The listing builds one solid part. Answer for the finished solid, in the listing's coordinates (mm). Give positions to 0.01 mm unless a question says otherwise; leave off trailing zeros. Loops run counter-clockwise (first coordinate to the right, second up) from the corner with the lowest first, then second, coordinate; pieces in that order, holes last. Notation, with made-up numbers: (42, 10) - (46, 10) arc R25 ccw to (46, 25) - close; hole circle Ø7 at (-34.75, -22). An arc over 180 degrees is marked (long way). Write each question's results on one line, items separated by ' | '.
from build123d import *
from build123d.topology import SkipClean

# Parameters (mm, degrees)
SKETCH1_R           = 2.98
BOSS_EXTRUDE1_DEPTH = 5.55
SKETCH2_R           = 2.5
CUT_EXTRUDE1_DEPTH  = 4.9
SKETCH3_R           = 1.44
CUT_EXTRUDE2_DEPTH  = 7.968737332
CHAMFER1_SIZE       = 0.25
THREAD1_PITCH       = 0.8


with BuildPart() as part:
    # Sketch1 → Boss-Extrude1 (new body)
    with BuildSketch(Plane(origin=(0, 0, 0), x_dir=(1, 0, 0), z_dir=(0, 1, 0))):
        with Locations(Location((0, 0, 0), (0, 0, 270))):
            Circle(SKETCH1_R)
    extrude(amount=BOSS_EXTRUDE1_DEPTH)

    # Sketch2 → Cut-Extrude1 (cut)
    with BuildSketch(Plane.XZ):
        with Locations(Location((0, 0, 0), (0, 0, 270))):
            Circle(SKETCH2_R)
    extrude(amount=-CUT_EXTRUDE1_DEPTH, mode=Mode.SUBTRACT)

    # Sketch3 → Cut-Extrude2 (cut, through all)
    with BuildSketch(Plane(origin=(0, 5.55, 0), x_dir=(1, 0, 0), z_dir=(0, 1, 0))):
        with Locations(Location((0, 0, 0), (0, 0, 270))):
            Circle(SKETCH3_R)
    extrude(amount=-CUT_EXTRUDE2_DEPTH, mode=Mode.SUBTRACT)

    # Chamfer1
    chamfer1_edges = [part.edges().sort_by_distance(p)[0] for p in [
        (0, 5.55, -2.98),
    ]]
    chamfer(chamfer1_edges, length=CHAMFER1_SIZE)

    # Thread1: the profile of Thread Profile1 profile screwed along a right-hand helix of 2.5 turns, 8 arcs to a turn; built about Z, then put on its axis
    with SkipClean():  # the faces are left unmerged after this step: merging them gives an invalid solid
        thread1_z = Axis((0, 0, 0), (0, 0, 1))
        thread1_corners = [(2.4997, 0, -0.000173205), (2.9330127, 0, 0.249999999), (2.9330127, 0, 0.349999999), (2.4997, 0, 0.600173203)]
        with BuildLine(mode=Mode.PRIVATE) as thread1_profile:
            Line(thread1_corners[0], thread1_corners[1])
            Line(thread1_corners[1], thread1_corners[2])
            Line(thread1_corners[2], thread1_corners[3])
            Line(thread1_corners[3], thread1_corners[0])
        thread1_cap = Face(thread1_profile.wire())
        thread1_turn_angles = [0, 22.5, 45, 67.5, 90, 112.5, 135, 157.5, 180, 202.5, 225, 247.5, 270, 292.5, 315, 337.5, 360]
        thread1_turn_weights = [1, 0.9238795325112867, 1, 0.9238795325112867, 1, 0.9238795325112867, 1, 0.9238795325112867, 1, 0.9238795325112867, 1, 0.9238795325112867, 1, 0.9238795325112867, 1, 0.9238795325112867, 1]
        thread1_turn_rails = [Edge.make_bspline([Vector(p[0], p[1], 0).rotate(thread1_z, thread1_turn_angles[k]) / thread1_turn_weights[k] + Vector(0, 0, p[2] + THREAD1_PITCH * thread1_turn_angles[k] / 360) for k in range(17)], [0, 0, 0, 1, 1, 2, 2, 3, 3, 4, 4, 5, 5, 6, 6, 7, 7, 8, 8, 8], 2, thread1_turn_weights) for p in thread1_corners]
        thread1_turn_sides = [Face.make_surface_from_curves(thread1_turn_rails[p[0]], thread1_turn_rails[p[1]]) for p in [(0, 1), (1, 2), (2, 3), (3, 0)]]
        thread1_last_angles = [720, 742.5, 765, 787.5, 810, 832.5, 855, 877.5, 900]
        thread1_last_weights = [1, 0.9238795325112867, 1, 0.9238795325112867, 1, 0.9238795325112867, 1, 0.9238795325112867, 1]
        thread1_last_rails = [Edge.make_bspline([Vector(p[0], p[1], 0).rotate(thread1_z, thread1_last_angles[k]) / thread1_last_weights[k] + Vector(0, 0, p[2] + THREAD1_PITCH * thread1_last_angles[k] / 360) for k in range(9)], [0, 0, 0, 1, 1, 2, 2, 3, 3, 4, 4, 4], 2, thread1_last_weights) for p in thread1_corners]
        thread1_last_sides = [Face.make_surface_from_curves(thread1_last_rails[p[0]], thread1_last_rails[p[1]]) for p in [(0, 1), (1, 2), (2, 3), (3, 0)]]
        thread1 = Plane(origin=(0, 0, 0), x_dir=(1, 0, 0), z_dir=(0, 1, 0)) * Solid(Shell([*[p.moved(Location((0, 0, THREAD1_PITCH * i))) for i in range(2) for p in thread1_turn_sides], *thread1_last_sides, thread1_cap, thread1_cap.rotate(thread1_z, 900).moved(Location((0, 0, THREAD1_PITCH * 900 / 360)))]))
        add(thread1, mode=Mode.SUBTRACT)


solid = part.part
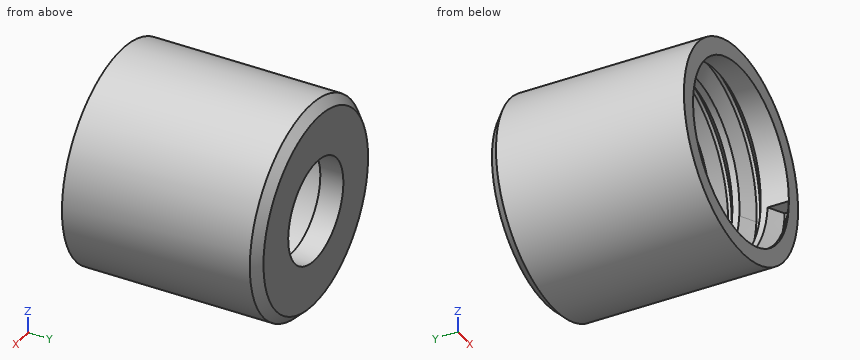
Item 1: A cutting plane is placed at A-A, the plane y = 4.25. Determine the outline of the cut face in (x, z).
Values found:
outline: circle Ø5.96 at (0, 0); hole circle Ø5 at (0, 0)
Item 2: Flat-ended cylindrical pins translate along their axes: P1, Ø1, axis at y = 1, z = -2, coming from the -X side; P2, Ø2, axis at y = 3.5, z = 2, coming from the -X side; P3, Ø0.5, axis at x = 2.5, y = 0.5, coming from the -Z side. Find the tip coordinate at first contact, or state that the pin passes through.
Values found:
P1: stops at x = -2.57 | P2: stops at x = -2.81 | P3: stops at z = -1.95
Item 3: Find the intervals of material crossed by line 1 along Y through (x, z) = (0, 2.7); line 2 along X through (y, z) = (3.65, 0.1); line 3 along Y through (x, z) = (-1.05, 1.3), in increasing order. Write a range as [from, to].
Values found:
line 1: y = [0, 0.72], [1.08, 1.52], [1.88, 5.55] | line 2: x = [-2.98, -2.5], [2.5, 2.98] | line 3: y = [4.9, 5.55]
